```python
from build123d import *

# Parameters (mm, degrees)
SKETCH1_R           = 10
BOSS_EXTRUDE1_DEPTH = 4.5
SKETCH2_R           = 10
SKETCH2_R_2         = 4.4
SKETCH2_R_3         = 2.75
CUT_EXTRUDE1_DEPTH  = 1.9
SKETCH4_R           = 1.75
CUT_EXTRUDE2_DEPTH  = 15.84082208
SKETCH5_R           = 2.75
CUT_EXTRUDE3_DEPTH  = 1


with BuildPart() as part:
    # Sketch1 → Boss-Extrude1 (new body)
    with BuildSketch(Plane(origin=(0, 0, 0), x_dir=(1, 0, 0), z_dir=(0, 1, 0))):
        with Locations(Location((0, 0, 0), (0, 0, 270))):
            Circle(SKETCH1_R)
    extrude(amount=BOSS_EXTRUDE1_DEPTH)

    # Sketch2 → Cut-Extrude1 (cut)
    # profile 1 of 2: a face of its own
    with BuildSketch(Plane.XZ):
        with Locations(Location((0, 0, 0), (0, 0, 270))):
            Circle(SKETCH2_R)
        with Locations(Location((0, 0, 0), (0, 0, 270))):
            Circle(SKETCH2_R_2, mode=Mode.SUBTRACT)
    # profile 2 of 2: a face of its own
    with BuildSketch(Plane.XZ):
        with Locations(Location((0, 0, 0), (0, 0, 270))):
            Circle(SKETCH2_R_3)
    extrude(amount=-CUT_EXTRUDE1_DEPTH, mode=Mode.SUBTRACT)

    # Sketch4 → Cut-Extrude2 (cut, through all)
    with BuildSketch(Plane(origin=(0, 4.5, 0), x_dir=(1, 0, 0), z_dir=(0, 1, 0))):
        with Locations(Location((0, 7, 0), (0, 0, 270))):
            Circle(SKETCH4_R)
        with Locations(Location((7, 0, 0), (0, 0, 270))):
            Circle(SKETCH4_R)
        with Locations(Location((0, -7, 0), (0, 0, 270))):
            Circle(SKETCH4_R)
        with Locations(Location((-7, 0, 0), (0, 0, 270))):
            Circle(SKETCH4_R)
    extrude(amount=-CUT_EXTRUDE2_DEPTH, mode=Mode.SUBTRACT)

    # Sketch5 → Cut-Extrude3 (cut)
    with BuildSketch(Plane.XZ.offset(-1.9)):
        with Locations(Location((0, 0, 0), (0, 0, 270))):
            Circle(SKETCH5_R)
    extrude(amount=-CUT_EXTRUDE3_DEPTH, mode=Mode.SUBTRACT)


solid = part.part
```
The listing builds one solid part. Answer for the finished solid, in the listing's coordinates (mm). A direction names the side the tool comes from. Coordinates: 2 decimals unless noted, no trailing zeros. Write each loop counter-clockwise with the first axis right and the second up, starting at its lowest first coordinate (ties: lowest second). Pieces come first, ordered by that corner, then holes. Notation, with made-up numbers: (66, 43.25) - (115, 43.25) arc R23 ccw to (115, 54.25) - close; hole circle Ø10 at (43, 58). An arc over 180 degrees is marked (long way). One line per item, written item: value.
1) Find section B-B (x = 0). Give the vertices of the cut face in (y, z), and give its area (3 significant figures).
Geometry check:
outline: (0, -4.4) - (1.9, -4.4) - (1.9, -5.25) - (4.5, -5.25) - (4.5, 5.25) - (1.9, 5.25) - (1.9, 4.4) - (0, 4.4) - (0, 2.75) - (2.9, 2.75) - (2.9, -2.75) - (0, -2.75) - close; (1.9, -10) - (4.5, -10) - (4.5, -8.75) - (1.9, -8.75) - close; (1.9, 8.75) - (4.5, 8.75) - (4.5, 10) - (1.9, 10) - close
area: 34.6 mm2
2) For a pull along Z with two mould halves and no side action, classify faces 3 (the cylindrical face through (-8.55, 3.22, 0.81)), 4 (the cylindrical face through (-9.76, 3.18, -2.17)), 5 (the flat face through (-2.1, 1.9, -4.3)) as pulls with the +Z half, pulls with the -Z half, needs draft (parallel to the pull), parting line crosses it, or undercut.
Geometry check:
face 3: undercut
face 4: parting line crosses it
face 5: needs draft
3) Each of these flat-tipped pins is pushed along its axis until it touches: pin 1 Ø2 at (x, y) = (-3, 1) entering from -Z; pin 2 Ø1.5 at (y, z) = (4, 1.5) entering from +X. Where does it stop, or does it pass through?
Geometry check:
pin 1: stops at z = -9.67
pin 2: stops at x = 9.97
4) A tool of negligible diameter and unlimited length cuts with its end or side. For faces 1 (the cylindrical face through (-2.685, 1.43, 0.596)), 2 (the cylindrical face through (-0.67, 3.218, -5.383)), from which of +Z, -Z, +X, -X, +Y, -Y can it reach the whole face along a straight path? Write none if from no direction.
Geometry check:
face 1: -Y
face 2: +Y, -Y
5) Find section C-C (y = 3.7). Give the vertices of the cut face in (x, z).
Geometry check:
outline: circle Ø20 at (0, 0); hole circle Ø3.5 at (-7, 0); hole circle Ø3.5 at (0, -7); hole circle Ø3.5 at (0, 7); hole circle Ø3.5 at (7, 0)
6) Consider line 1 along X through (y, z) = (4, 0); line 2 along X through (y, z) = (2.2, -1); line 3 along Z through (x, y) = (1.25, 1.95). Determine where each line is inside the solid, lowest interval first. Write a range as from..to.
Geometry check:
line 1: x = -10..-8.75, -5.25..5.25, 8.75..10
line 2: x = -9.95..-8.44, -5.56..-2.56, 2.56..5.56, 8.44..9.95
line 3: z = -9.92..-8.22, -5.78..-2.45, 2.45..5.78, 8.22..9.92
7) Find section A-A (z = 0). Give the vertices of the cut face in (x, y), and give its area (3 significant figures).
Geometry check:
outline: (-10, 1.9) - (-8.75, 1.9) - (-8.75, 4.5) - (-10, 4.5) - close; (-5.25, 1.9) - (-4.4, 1.9) - (-4.4, 0) - (-2.75, 0) - (-2.75, 2.9) - (2.75, 2.9) - (2.75, 0) - (4.4, 0) - (4.4, 1.9) - (5.25, 1.9) - (5.25, 4.5) - (-5.25, 4.5) - close; (8.75, 1.9) - (10, 1.9) - (10, 4.5) - (8.75, 4.5) - close
area: 34.6 mm2
8) Find section D-D (z = -7.5). Give the vertices of the cut face in (x, y).
Geometry check:
outline: (-6.61, 1.9) - (-1.68, 1.9) - (-1.68, 4.5) - (-6.61, 4.5) - close; (1.68, 1.9) - (6.61, 1.9) - (6.61, 4.5) - (1.68, 4.5) - close
